The listing builds one solid part. Answer for the finished solid, in the listing's coordinates (mm). A direction names the side the tool comes from. Coordinates: 2 decimals unless noted, no trailing zeros. Write each loop counter-clockwise with the first axis right and the second up, starting at its lowest first coordinate (ties: lowest second). Pieces come first, ordered by that corner, then holes. Notation, with made-up numbers: M -14,-13.5 L 12,-13.5 A35 ccw 12,21.5 Z; hole C -36.5,51 d9. An arc over 180 degrees is marked long. Answer as CSV lines item,"result".
```python
from build123d import *

# Parameters (mm, degrees)
F1_DEPTH = 508
F3_DEPTH = 635
F4_R     = 381
F5_DEPTH = 1143


with BuildPart() as f1:
    # F0 (on Top) → F1 (new body)
    with BuildSketch(Plane.XY):
        with BuildLine():
            Line((-762, -508), (762, -508))
            ThreePointArc((762, -508), (1270, 0), (762, 508))
            Line((762, 508), (-762, 508))
            Line((-762, 508), (-762, 254))
            Line((-762, 254), (-381, 254))
            ThreePointArc((-381, 254), (-127, 0), (-381, -254))
            Line((-381, -254), (-762, -254))
            Line((-762, -254), (-762, -508))
        make_face()
    extrude(amount=F1_DEPTH)

    # F2 (on face) → F3 (join)
    with BuildSketch(Plane.XY.offset(508)):
        with BuildLine():
            ThreePointArc((762, -508), (1121.210245, -359.210245), (1270, 0))
            ThreePointArc((1270, 0), (1121.210245, 359.210245), (762, 508))
            ThreePointArc((762, 508), (254, 0), (762, -508))
        make_face()
    extrude(amount=F3_DEPTH)

    # F4 (on face) → F5 (cut)
    with BuildSketch(Plane.XY.offset(1143)):
        with Locations((762, 0)):
            Circle(F4_R)
    extrude(amount=-F5_DEPTH, mode=Mode.SUBTRACT)


solid = f1.part
```
Q1. Find section A-A (x = -413). Give the vertices of the cut face in (y, z), and give its area (3 significant figures).
Output:
outline,"M -508,0 L -254,0 L -254,508 L -508,508 Z; M 254,0 L 508,0 L 508,508 L 254,508 Z"
area,"258,000 mm2"
Q2. Find section D-D (x = 1030.5). Give the vertices of the cut face in (y, z), and give its area (3 significant figures).
Output:
outline,"M -431.24,0 L -270.31,0 L -270.31,1143 L -431.24,1143 Z; M 270.31,0 L 431.24,0 L 431.24,1143 L 270.31,1143 Z"
area,"368,000 mm2"
Q3. Flat-ended cylindrical pins translate along their axes: pin 1 Ø4 at (x, z) = (976.5, 991.5) entering from -Y; pin 2 Ø1 at (y, z) = (-54, 444) entering from -X; pin 3 Ø6 at (y, z) = (331.5, 325) entering from +X. Find the tip coordinate at first contact, or state that the pin passes through.
Output:
pin 1,"y = -461.42"
pin 2,"x = -132.92"
pin 3,"x = 1149.49"
Q4. Find section C-C (y = -83). Give the vertices of the cut face in (x, z).
Output:
outline,"M -140.94,0 L 390.15,0 L 390.15,1143 L 260.83,1143 L 260.83,508 L -140.94,508 Z; M 1133.85,0 L 1263.17,0 L 1263.17,1143 L 1133.85,1143 Z"
Q5. The mould has two halves that part along Y. Classify faces 1 (the flat face through (11, 508, 250)), 2 (the flat face through (-11, 7, 508)), 3 (the cylindrical face through (459.65, -231.83, 579.5)): pulls with the +Y half, pulls with the -Y half, needs draft (parallel to the pull), parting line crosses it, or undercut.
Output:
face 1,"pulls with the +Y half"
face 2,"needs draft"
face 3,"undercut"
Q6. For faces 4 (the flat face through (-11, -508, 250)), 5 (the flat face through (-574, 254, 250)), determine the directions among +Z, -Z, +X, -X, +Y, -Y from which every point of the face is accessible in a straight line to the end or side of a thin tool.
Output:
face 4,"+Z, -Z, +X, -X, -Y"
face 5,"+Z, -Z, -X"
Q7. Straight lines are drawn through the part: line 1 (Y direction, x = 762, z = 715.5); line 2 (Y direction, x = -399.5, z = 460); line 3 (X direction, y = 263.5, z = 454.5). For each, find the intervals that lie inside material, in ascending order.
Output:
line 1,"-508 to -381, 381 to 508"
line 2,"-508 to -254, 254 to 508"
line 3,"-762 to 486.81, 1037.19 to 1196.32"
Q8. Find section B-B (z = 151). Give the vertices of the cut face in (x, y).
Output:
outline,"M -762,-508 L 762,-508 A508 ccw 762,508 L -762,508 L -762,254 L -381,254 A254 cw -381,-254 L -762,-254 Z; hole C 762,0 d762"
